Autodesk Inventor part; units mm, degrees
ref_plane "YZ Plane" through (0, 0, 0) normal (1, 0, 0) x (0, 1, 0)
ref_plane "XZ Plane" through (0, 0, 0) normal (0, 1, 0) x (-1, 0, 0)
ref_plane "XY Plane" through (0, 0, 0) normal (0, 0, 1) x (1, 0, 0)
sketch "Boceto1" plane through (0, 0, 0) normal (0, 1, 0) x (-1, 0, 0)
  line L0 (0, 0) -> (0, -350)
  line L1 (0, -350) -> (-350, 0)
  line L2 (-350, 0) -> (0, 0)
  dimension "d0" = 350
  dimension "d1" = 45
extrude "Extrusión1" add sketch "Boceto1" along normal blind 1
sketch "Boceto2" plane through (0, 1, 0) normal (0, 1, 0) x (1, 0, 0)
  line L0 (350, 0) -> (0, 350)
  line L1 (350, 0) -> (349, 0)
  line L2 (0, 0) -> (350, 0)
  line L3 (0, 350) -> (0, 349)
  line L4 (0, 350) -> (0, 0)
  line L5 (0, 0) -> (0, 1)
  line L6 (0, 0) -> (1, 0)
  line L7 (349, 0) -> (0, 349)
  line L8 (1, 0) -> (1, 348)
  line L9 (0, 1) -> (348, 1)
  dimension "d4" = 1
  dimension "d5" = 1
  dimension "d6" = 1
  dimension "d7" = 1
extrude "Extrusión2" add sketch "Boceto2" along normal blind 348 contours L1 L7 L3 L0 | L2 L8 L9 L7 | L2 L4 L9 L8
sketch "Boceto3" plane through (0, 349, 0) normal (0, 1, 0) x (1, 0, 0)
  line L0 (0, 350) -> (0, 0)
  line L1 (0, 0) -> (0, 350)
  line L2 (0, 0) -> (350, 0)
  line L3 (0, 350) -> (350, 0)
  line L4 (350, 0) -> (0, 0)
extrude "Extrusión3" add sketch "Boceto3" along normal blind 1
sketch "Boceto4" plane through (0, 0, -350) normal (-1, 0, 0) x (0, 0, 1)
  line L0 (349, 1) -> (349, 349)
  line L1 (349, 1) -> (349, 349)
  line L2 (1, 1) -> (1, 349)
  line L3 (349, 349) -> (1, 349)
  line L4 (1, 349) -> (1, 1)
  line L5 (1, 1) -> (349, 1)
  line L6 (0, 0) -> (0, 350)
  line L7 (0, 350) -> (350, 350)
  line L8 (350, 0) -> (350, 350)
  line L9 (350, 350) -> (350, 0)
  line L10 (350, 0) -> (0, 0)
  line L11 (350, 0) -> (0, 0)
  line L12 (0, 0) -> (0, 350)
extrude "Extrusión4" add sketch "Boceto4" along normal blind 233.1
properties part number "cajon_1_proyecto_diseno"
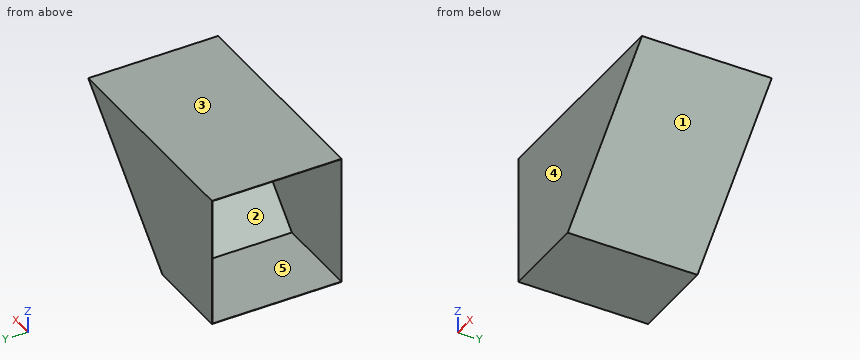
Geometry check sheet. Reference: the model listing, model coordinates, mm. Face numbers are marked on the shaded views. A direction names the side the tool comes from. Coordinates: 2 decimals unless noted, no trailing zeros. Order: outer loops, then holes, each group sorted by start corner. A loop starts at its lowest first (then second) coordinate and runs counter-clockwise, first axis right, second up.
Item 1: Section check D-D (x = -51). Enter the section's corners in (y, z).
Item 2: Scan lines: line 1 along Y through (x, z) = (58.5, -153); line 2 along Z through (x, y) = (-196, 115); line 3 along Z through (x, y) = (217, 120). Record each from-to range of solid material in increasing order.
Item 3: Depth check by flat-ended pin: pin 1 (5 mm diameter, centred on y = 42.5, z = -122.5, fed in from -X); pin 2 (2 mm diameter, centred on y = 240, z = -202.5, fed in from +X); pin 3 (2 mm diameter, centred on y = 36.5, z = -217.5, fed in from +X). Enter the tip coordinate at first touch or a pass-through.
Item 4: Section check C-C (y = 190). Enter the section's corners in (x, z), plus the area to 3 significant figures.
Item 5: Mould release check, pull along Y, two halves, no side actions. Record for the marked faces 3, 4 and 5: released by +Y, released by -Y, zero draft, split by the parting line, or undercut.
Item 6: Section check A-A (x = 31). Enter the section's corners in (y, z), plus the area to 3 significant figures.
Item 7: Section check B-B (z = -64.5). Enter the section's corners in (x, y), plus the area to 3 significant figures.
Item 8: Tool access check on the marked faces 1 and 2. Record the directions out of +Z, -Z, +X, -X, +Y, -Y that give a thin tool (end or side, any length) a straight path to the whole face; none if there is none.
Check sheet entries:
1. outline: (0, -350) - (350, -350) - (350, 0) - (0, 0) - close; hole (1, -349) - (349, -349) - (349, -1) - (1, -1) - close
2. line 1: y = 0 to 1, 349 to 350
2. line 2: z = -350 to -349, -1 to 0
2. line 3: z = -133 to -132, -1 to 0
3. pin 1: stops at x = 224
3. pin 2: stops at x = 148.5
3. pin 3: stops at x = 133.5
4. outline: (-233.1, -350) - (0, -350) - (350, 0) - (-233.1, 0) - (-233.1, -1) - (348, -1) - (0, -349) - (-233.1, -349) - close
4. area: 1,160 mm2
5. face 3: zero draft
5. face 4: released by -Y
5. face 5: undercut
6. outline: (0, -319) - (350, -319) - (350, 0) - (0, 0) - close; hole (1, -318) - (349, -318) - (349, -1) - (1, -1) - close
6. area: 1,330 mm2
7. outline: (-233.1, 0) - (285.5, 0) - (285.5, 350) - (-233.1, 350) - (-233.1, 349) - (284.5, 349) - (284.5, 1) - (-233.1, 1) - close
7. area: 1,390 mm2
8. face 1: -Z, +X, +Y, -Y
8. face 2: -X
